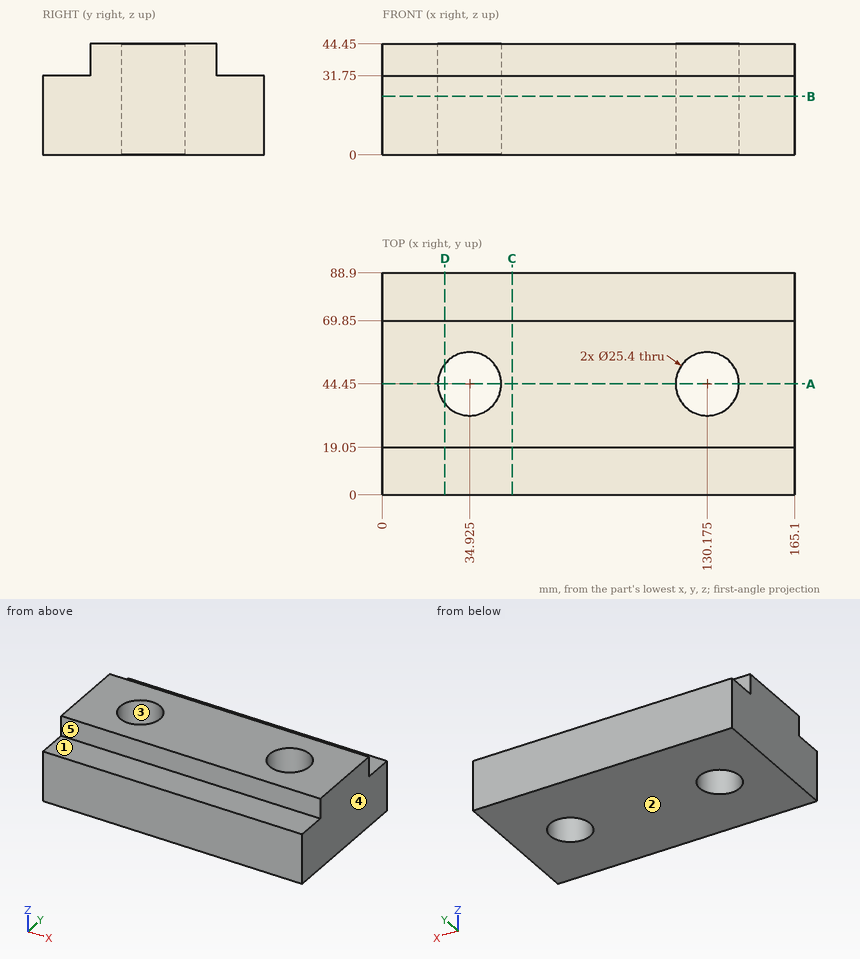
Can you work these out from the drawing? Everything is in mm from the part's minimum corner. A direction names the side the tool comes from. Coordinates: 2 decimals unless noted, no trailing zeros. Loops run counter-clockwise (first coordinate to the right, second up) from the corner with the lowest first, then second, coordinate; pieces in that order, holes last. Notation, with made-up numbers: (-11.75, 0.25) -> (39.25, 0.25) arc R33 cw to (39.25, 29.25) -> close; hole circle Ø6 at (10, -38). An arc over 180 degrees is marked (long way). Return JSON: item names as keys, results as strings.
1) Will these pins go through, and if not, where does the flat tip stop? pin 1 (20.5 mm diameter, centred on x = 34.925, y = 44.45, fed in from -Z); pin 2 (4 mm diameter, centred on x = 84.5, z = 38, fed in from -Y); pin 3 (6.5 mm diameter, centred on x = 112, z = 39.5, fed in from +Y); pin 4 (9.5 mm diameter, centred on x = 81, y = 76, fed in from +Z).
Results below:
{"pin 1": "through", "pin 2": "y = 19.05", "pin 3": "y = 69.85", "pin 4": "z = 31.75"}
2) If we section it at C-C, the plane x = 52: Write out the boundary of the cut face in (y, z).
Results below:
{"outline": "(0, 0) -> (88.9, 0) -> (88.9, 31.75) -> (69.85, 31.75) -> (69.85, 44.45) -> (19.05, 44.45) -> (19.05, 31.75) -> (0, 31.75) -> close"}
3) For the marked faces 1 and 2, which set-ups out of +Z, -Z, +X, -X, +Y, -Y let a thin tool reach every point of the face, with its end or its side?
Results below:
{"face 1": "+Z, +X, -X, -Y", "face 2": "-Z, +X, -X, +Y, -Y"}
4) If we section it at A-A, the plane y = 44.45: Write out the boundary of the cut face in (x, z) (3 decimals), then the cut area to 3 significant figures.
Results below:
{"outline": "(0, 0) -> (22.225, 0) -> (22.225, 44.45) -> (0, 44.45) -> close; (47.625, 0) -> (117.475, 0) -> (117.475, 44.45) -> (47.625, 44.45) -> close; (142.875, 0) -> (165.1, 0) -> (165.1, 44.45) -> (142.875, 44.45) -> close", "area": "5,080 mm²"}
5) If we section it at B-B, the plane z = 23.5: Write out the boundary of the cut face in (x, y) (3 decimals).
Results below:
{"outline": "(0, 0) -> (165.1, 0) -> (165.1, 88.9) -> (0, 88.9) -> close; hole circle Ø25.4 at (34.925, 44.45); hole circle Ø25.4 at (130.175, 44.45)"}
6) If we section it at D-D, the plane x = 25: Write out the boundary of the cut face in (y, z), then the cut area to 3 significant figures.
Results below:
{"outline": "(0, 0) -> (36.53, 0) -> (36.53, 44.45) -> (19.05, 44.45) -> (19.05, 31.75) -> (0, 31.75) -> close; (52.37, 0) -> (88.9, 0) -> (88.9, 31.75) -> (69.85, 31.75) -> (69.85, 44.45) -> (52.37, 44.45) -> close", "area": "2,760 mm²"}
7) I need wall thicknesses on line 1 (X direction, y = 44, z = 23); line 2 (X direction, y = 37, z = 6); line 3 (Z direction, x = 59, y = 83). Which ranges of each line are inside material? Lowest first, please. Write a range as from..to.
Results below:
{"line 1": "0..22.23, 47.62..117.48, 142.87..165.1", "line 2": "0..24.64, 45.21..119.89, 140.46..165.1", "line 3": "0..31.75"}
8) Thinking about a two-plate mould opening in X: for the marked faces 3, 4 and 5, which applies, +X half, -X half, draft (parallel to the pull), parting line (faces both ways), or undercut?
Results below:
{"face 3": "undercut", "face 4": "+X half", "face 5": "draft"}
